```python
from build123d import *

# Parameters (mm, degrees)
SKETCH_AS_DRAWN_R                   = 2.25
EXTRUDE_DEPTH                       = 10
EXTRUDE_ONTO_SKETCH_ROLL_ANGLE      = 90
EXTRUDE_ONTO_SKETCH_PLACEMENT_ANGLE = 180
BOX_W                               = 72
BOX_H                               = 3
BOX_DEPTH                           = 210
SKETCH001_R                         = 1.65
HOLE_DEPTH                          = 25
SKETCH002_R                         = 1.65
HOLE001_DEPTH                       = 3.001
SKETCH004_R                         = 6
HOLE002_DEPTH                       = 25


with BuildPart() as extrude_body:
    # Sketch as drawn → Extrude (new)
    with BuildSketch(Plane.XY):
        with Locations((-6, 4)):
            Circle(SKETCH_AS_DRAWN_R)
        with Locations((-66, 4)):
            Circle(SKETCH_AS_DRAWN_R)
        with Locations((-36, 4)):
            Circle(SKETCH_AS_DRAWN_R)
    extrude(amount=-EXTRUDE_DEPTH)


with BuildPart() as extrude_body_1:
    # Extrude onto Sketch roll: moved
    add(extrude_body.part.rotate(Axis((0, 0, 0), (1, 0, 0)), EXTRUDE_ONTO_SKETCH_ROLL_ANGLE))


with BuildPart() as extrude_body_2:
    # Extrude onto Sketch placement: moved
    add(extrude_body_1.part.moved(Location((0, 3, 0))).rotate(Axis((0, 3, 0), (0, 0, 1)), EXTRUDE_ONTO_SKETCH_PLACEMENT_ANGLE))


with BuildPart() as part_mirroring:
    # Part__Mirroring: instance of Extrude body
    add(extrude_body_2.part.mirror(Plane(origin=(0, 0, 105), x_dir=(0, 1, 0), z_dir=(0, 0, 1))))


with BuildPart() as fusion:
    # Fusion base: copy of Extrude body
    add(extrude_body_2.part)

    # Fusion: union Part__Mirroring
    add(part_mirroring.part)


with BuildPart() as body:
    # Box → Box (new body)
    with BuildSketch(Plane.XY):
        with Locations((36, 1.5)):
            Rectangle(BOX_W, BOX_H)
    extrude(amount=BOX_DEPTH)

    # Cut: cut Fusion
    add(fusion.part, mode=Mode.SUBTRACT)

    # Sketch001 (on Face2 of BaseFeature) → Hole (cut)
    with BuildSketch(Plane.XZ):
        with Locations((67, 50)):
            Circle(SKETCH001_R)
        with Locations((5, 50)):
            Circle(SKETCH001_R)
        with Locations((67, 92)):
            Circle(SKETCH001_R)
        with Locations((5, 92)):
            Circle(SKETCH001_R)
        with Locations((67, 154)):
            Circle(SKETCH001_R)
        with Locations((5, 154)):
            Circle(SKETCH001_R)
        with Locations((5, 112)):
            Circle(SKETCH001_R)
        with Locations((67, 112)):
            Circle(SKETCH001_R)
        with Locations((5, 164)):
            Circle(SKETCH001_R)
        with Locations((67, 164)):
            Circle(SKETCH001_R)
    extrude(amount=-HOLE_DEPTH, mode=Mode.SUBTRACT)

    # Sketch002 (on Face4 of Hole) → Hole001 (cut, through all)
    with BuildSketch(Plane(origin=(0, 3, 0), x_dir=(-1, 0, 0), z_dir=(0, 1, 0))):
        with Locations((-36, 35)):
            Circle(SKETCH002_R)
        with Locations((-20.5, 28)):
            Circle(SKETCH002_R)
        with Locations((-28.25, 41.423394)):
            Circle(SKETCH002_R)
        with Locations((-43.75, 41.423394)):
            Circle(SKETCH002_R)
        with Locations((-43.75, 14.576606)):
            Circle(SKETCH002_R)
        with Locations((-28.25, 14.576606)):
            Circle(SKETCH002_R)
        with Locations((-51.5, 28)):
            Circle(SKETCH002_R)
    extrude(amount=-HOLE001_DEPTH, mode=Mode.SUBTRACT)

    # Sketch004 (on Face2 of Hole001) → Hole002 (cut)
    with BuildSketch(Plane.XZ):
        with Locations((36, 35)):
            Circle(SKETCH004_R)
    extrude(amount=-HOLE002_DEPTH, mode=Mode.SUBTRACT)


solid = body.part
```
Can you work these out from the model? Positions are in its coordinate system, mm. Round coordinates to 2 decimals unless told otherwise and drop trailing zeros. Order: outer loops, then holes, each group sorted by start corner. A loop starts at its lowest first (then second) coordinate and runs counter-clockwise, first axis right, second up.
(1) I'm going to push flat-ended pins straight in: pin 1 (4 mm diameter, centred on x = 36, z = 4, fed in from +Y); pin 2 (6 mm diameter, centred on x = 6, z = 4, fed in from -Y). Where does each tip first touch, or does it pass through?
Results are:
pin 1: passes through
pin 2: stops at y = 0
(2) If I drill on L1, parallel to X at y = 1.8, z = 206; L2, parallel to X at y = 0.7, z = 164; L3, parallel to Z at x = 38, y = 0.95, over which ranges is the centre line in solid material (lowest first)?
Results are:
L1: x = 0 to 3.75, 8.25 to 33.75, 38.25 to 63.75, 68.25 to 72
L2: x = 0 to 3.35, 6.65 to 65.35, 68.65 to 72
L3: z = 0 to 2.97, 5.03 to 29.34, 40.66 to 204.97, 207.03 to 210
(3) If we section it at A-A (x = 36): Please give me the cut outline in (y, z), plus the area to 3 significant figures.
Results are:
outline: (0, 0) - (3, 0) - (3, 1.75) - (0, 1.75) - close; (0, 6.25) - (3, 6.25) - (3, 29) - (0, 29) - close; (0, 41) - (3, 41) - (3, 203.75) - (0, 203.75) - close; (0, 208.25) - (3, 208.25) - (3, 210) - (0, 210) - close
area: 567 mm2
(4) We'd pull the mould along Z, two halves only. Please class faces 1 (the face through (35, 0, 104)), 2 (the face through (68.248, 1.521, 4.099)): +Z half, -Z half, draft (parallel to the pull), parting line (faces both ways), or undercut.
Results are:
face 1: draft
face 2: undercut
(5) If we section it at B-B (z = 206): Please give me the cut outline in (x, y).
Results are:
outline: (0, 0) - (3.75, 0) - (3.75, 3) - (0, 3) - close; (8.25, 0) - (33.75, 0) - (33.75, 3) - (8.25, 3) - close; (38.25, 0) - (63.75, 0) - (63.75, 3) - (38.25, 3) - close; (68.25, 0) - (72, 0) - (72, 3) - (68.25, 3) - close
(6) If we section it at C-C (y = 2.2): Count the separate pieces of the cut face and the enclosed holes in it, plus the area to 3 significant figures.
Results are:
separate pieces: 1
enclosed holes: 23
area: 14,800 mm2
